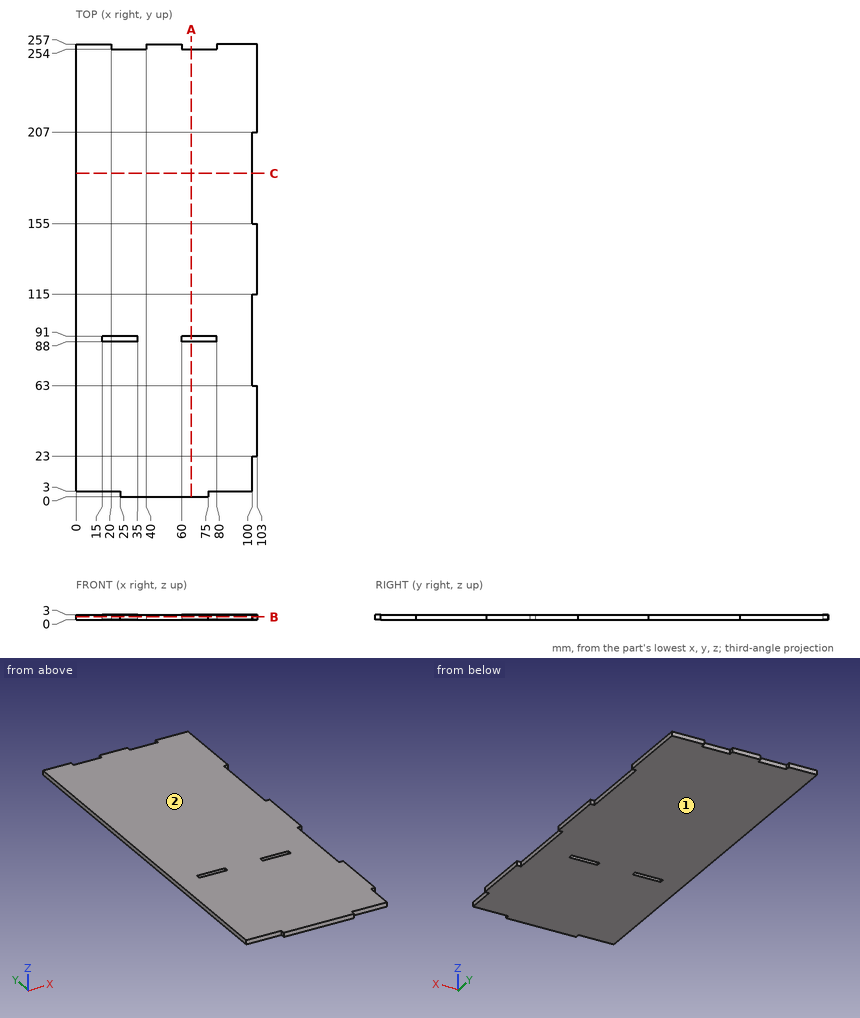
Verification items for this drawing (mm, ordinates from the low corner). Round coordinates to 2 decimals unless told otherwise and drop trailing zeros. Write each loop counter-clockwise with the first axis right and the second up, starting at its lowest first coordinate (ties: lowest second). Pieces come first, ordered by that corner, then holes. Notation, with made-up numbers: M 61,-1.75 L 115,-1.75 A22 ccw 115,18.25 Z; hole C 37.5,75.5 d3. An arc over 180 degrees is marked long. Write item = value, one per line. Start each with the question number.
1. Section check A-A, the plane x = 65.5. Record the cut outline in (y, z), then the cut area to 3 significant figures.
2. Gauge pin test, flat ends, axial feed: pin 1 (1.5 mm diameter, centred on y = 88, z = 2.5, fed in from +X); pin 2 (0.9 mm diameter, centred on x = 25.5, z = 1.5, fed in from +Y); pin 3 (8 mm diameter, centred on x = 72.5, y = 127, fed in from -Z); pin 4 (0.9 mm diameter, centred on x = 102, z = 1.5, fed in from -Y). Record the tip position at first contact, or that the pin passes through.
3. Release check for a two-part mould opening along Z. For the marked faces 1 and 2 record: pulls with the +Z half, pulls with the -Z half, needs draft (parallel to the pull), parting line crosses it, or undercut.
4. Section check B-B, the plane z = 1.65. State how many separate pieces and enclosed holes the cut face has, then the cut area to 3 significant figures.
5. Scan lines: line 1 (Y direction, x = 63, z = 1.15); line 2 (Y direction, x = 23.5, z = 0.9); line 3 (X direction, y = 81, z = 0.45). Record each from-to range of solid material in increasing order. Write a range as [from, to].
6. Section check C-C, the plane y = 183.5. Record the cut outline in (x, z).
Results found:
q1.outline = M 0,0 L 88,0 L 88,3 L 0,3 Z; M 91,0 L 254,0 L 254,3 L 91,3 Z
q1.area = 753 mm^2
q2.pin_1 = 100
q2.pin_2 = 254
q2.pin_3 = 0
q2.pin_4 = 23
q3.face_1 = pulls with the -Z half
q3.face_2 = pulls with the +Z half
q4.separate_pieces = 1
q4.enclosed_holes = 2
q4.area = 25,700 mm^2
q5.line_1 = [0, 88], [91, 254]
q5.line_2 = [3, 88], [91, 254]
q5.line_3 = [0, 100]
q6.outline = M 0,0 L 100,0 L 100,3 L 0,3 Z
